Geometry: final body of the model. Coordinates: model frame, mm. A direction names the side the tool comes from. Round coordinates to 2 decimals unless told otherwise and drop trailing zeros. Loops run counter-clockwise (first coordinate to the right, second up) from the corner with the lowest first, then second, coordinate; pieces in that order, holes last. Notation, with made-up numbers: (56, -38.75) - (87, -38.75) arc R4 ccw to (87, -31.75) - close; hole circle Ø6 at (-11.5, -24.75). An arc over 180 degrees is marked (long way). Answer as a JSON object with one key per item and string values. Group by question number.
Item 1: First-contact query: pin 1 (7.5 mm diameter, centred on x = 0, y = 0, fed in from +Z). Flat tip, straight axial feed; report the tip coordinate or a pass-through.
Item 2: Section B-B (x = 0). Return the cut outline in (y, z), plus the area to 3 significant figures.
Item 3: Reachability of faces 4 (the face through (0, -15.65, 1)), 5 (the face through (2.4, -2.4, -2.9)) from +Z, -Z, +X, -X, +Y, -Y: full face, straight path, thin tool, end or side. Return the list, or none.
Item 4: Draft query along X for faces 1 (the face through (-2.947, -0.13, -3.711)), 2 (the face through (20.05, 0, -1)), 3 (the face through (0, 4, -4.5)). Return one class per face: released by +X, released by -X, zero draft, split by the parting line, or undercut.
Item 5: Line query: line 1 (Y direction, x = 0, z = -3.95); line 2 (X direction, y = 0, z = -3.4); line 3 (Y direction, x = 0, z = 2.25). Output: solid intervals per line, ascending.
Item 6: Section C-C (z = 0). Return the cut outline in (x, y).
Item 7: Section D-D (y = 6.5). Return the cut outline in (x, z), plus the area to 3 significant figures.
Item 8: Section A-A (y = 0). Return the cut outline in (x, z).
```python
from build123d import *

# Parameters (mm, degrees)
F0_W      = 40.1
F0_H      = 31.3
F1_DEPTH  = 2.65
F2_W      = 34
F2_H      = 31.3
F3_DEPTH  = 2.85
F5_DEPTH  = 31.3
F6_DEPTH  = 4.5
F7_R      = 2.95
F8_DEPTH  = 25
F9_R      = 5.5
F9_R_2    = 2.95
F10_DEPTH = 8.4


with BuildPart() as f1:
    # F0 (on Top) → F1 (new body)
    with BuildSketch(Plane.XY):
        Rectangle(F0_W, F0_H)
    extrude(amount=F1_DEPTH)

    # F2 (on face) → F3 (join)
    with BuildSketch(Plane.XY.offset(2.65)):
        Rectangle(F2_W, F2_H)
    extrude(amount=F3_DEPTH)

    # F4 (on face) → F5 (join)
    with BuildSketch(Plane.XZ.offset(15.65)):
        Polygon((20.05, 2.65), (17, 5.5), (17, 2.65), align=None)
        Polygon((-17, 5.5), (-20.05, 2.65), (-17, 2.65), align=None)
    extrude(amount=-F5_DEPTH)

    # F6 (add): a face of the model
    f6_faces = [f1.faces().sort_by_distance(p)[0] for p in [
        (0, 0, 0),
    ]]
    extrude(f6_faces, amount=F6_DEPTH)

    # F7 (on face) → F8 (cut)
    with BuildSketch(Plane(origin=(0, 0, -4.5), x_dir=(1, 0, 0), z_dir=(0, 0, -1))):
        Circle(F7_R)
    extrude(amount=-F8_DEPTH, mode=Mode.SUBTRACT)

    # F9 (on face) → F10 (cut)
    with BuildSketch(Plane.XY.offset(5.5)):
        Circle(F9_R)
        Circle(F9_R_2, mode=Mode.SUBTRACT)
    extrude(amount=-F10_DEPTH, mode=Mode.SUBTRACT)


solid = f1.part
```
Values:
{
 "1": {"pin 1": "stops at z = -2.9"},
 "2": {"outline": "(-15.65, -4.5) - (-2.95, -4.5) - (-2.95, -2.9) - (-5.5, -2.9) - (-5.5, 5.5) - (-15.65, 5.5) - close; (2.95, -4.5) - (15.65, -4.5) - (15.65, 5.5) - (5.5, 5.5) - (5.5, -2.9) - (2.95, -2.9) - close", "area": "211 mm^2"},
 "3": {"face 4": "+Z, -Z, +X, -X, -Y", "face 5": "+Z"},
 "4": {"face 1": "undercut", "face 2": "released by +X", "face 3": "zero draft"},
 "5": {"line 1": "y = -15.65 to -2.95, 2.95 to 15.65", "line 2": "x = -20.05 to -2.95, 2.95 to 20.05", "line 3": "y = -15.65 to -5.5, 5.5 to 15.65"},
 "6": {"outline": "(-20.05, -15.65) - (20.05, -15.65) - (20.05, 15.65) - (-20.05, 15.65) - close; hole circle Ø11 at (0, 0)"},
 "7": {"outline": "(-20.05, -4.5) - (20.05, -4.5) - (20.05, 2.65) - (17, 5.5) - (-17, 5.5) - (-20.05, 2.65) - close", "area": "392 mm^2"},
 "8": {"outline": "(-20.05, -4.5) - (-2.95, -4.5) - (-2.95, -2.9) - (-5.5, -2.9) - (-5.5, 5.5) - (-17, 5.5) - (-20.05, 2.65) - close; (2.95, -4.5) - (20.05, -4.5) - (20.05, 2.65) - (17, 5.5) - (5.5, 5.5) - (5.5, -2.9) - (2.95, -2.9) - close"}
}
